Verification items for the finished model (mm, model axes). Coordinates: 2 decimals unless noted, no trailing zeros. Write each loop counter-clockwise with the first axis right and the second up, starting at its lowest first coordinate (ties: lowest second). Pieces come first, ordered by that corner, then holes. Notation, with made-up numbers: (2.5, 79.5) -> (60.5, 79.5) arc R28 cw to (60.5, 102.5) -> close; hole circle Ø6 at (-21.75, 78.5). An arc over 180 degrees is marked (long way). Answer in a Markdown table with one row per item.
```python
from build123d import *

# Parameters (mm, degrees)
SKETCH_W     = 42.3
SKETCH_H     = 42.3
SKETCH_R     = 11
PAD_DEPTH    = 2
CHAMFER_SIZE = 3.535534
SKETCH001_R  = 1.5
POCKET_DEPTH = 2.001


with BuildPart() as part:
    # Sketch → Pad (new body)
    with BuildSketch(Plane.XY):
        Rectangle(SKETCH_W, SKETCH_H)
        Circle(SKETCH_R, mode=Mode.SUBTRACT)
    extrude(amount=PAD_DEPTH)

    # Chamfer
    chamfer_edges = [part.edges().sort_by_distance(p)[0] for p in [
        (21.15, -21.15, 1),
        (21.15, 21.15, 1),
        (-21.15, -21.15, 1),
        (-21.15, 21.15, 1),
    ]]
    chamfer(chamfer_edges, length=CHAMFER_SIZE)

    # Sketch001 (on Face5 of Chamfer) → Pocket (cut, through all)
    with BuildSketch(Plane.XY.offset(2)):
        with Locations((15.5, 15.5)):
            Circle(SKETCH001_R)
        with Locations((-15.5, -15.5)):
            Circle(SKETCH001_R)
        with Locations((15.5, -15.5)):
            Circle(SKETCH001_R)
        with Locations((-15.5, 15.5)):
            Circle(SKETCH001_R)
    extrude(amount=-POCKET_DEPTH, mode=Mode.SUBTRACT)


solid = part.part
```
1. Sectioned sample at C-C, the plane z = 1.35. Record the cut outline in (x, y).
Findings below:
| item | result |
|---|---|
| outline | (-21.15, -17.61) -> (-17.61, -21.15) -> (17.61, -21.15) -> (21.15, -17.61) -> (21.15, 17.61) -> (17.61, 21.15) -> (-17.61, 21.15) -> (-21.15, 17.61) -> close; hole circle Ø3 at (-15.5, -15.5); hole circle Ø3 at (-15.5, 15.5); hole circle Ø22 at (0, 0); hole circle Ø3 at (15.5, -15.5); hole circle Ø3 at (15.5, 15.5) |
2. Release check for a two-part mould opening along X. For faces 1 (the face through (-10, -9, 0)), 2 (the face through (-2.38, -10.74, 0.99)), 3 (the face through (-19.357, -19.407, 0.986)) record: released by +X, released by -X, zero draft, split by the parting line, or undercut.
Findings below:
| item | result |
|---|---|
| face 1 | zero draft |
| face 2 | undercut |
| face 3 | released by -X |
3. Sectioned sample at B-B, the plane y = 0. Record the cut outline in (x, z).
Findings below:
| item | result |
|---|---|
| outline | (-21.15, 0) -> (-11, 0) -> (-11, 2) -> (-21.15, 2) -> close; (11, 0) -> (21.15, 0) -> (21.15, 2) -> (11, 2) -> close |
4. Material ranges on probe 1 along Y at (x, z) = (15.5, 1.6); probe 2 along X at (y, z) = (16, 1.05); probe 3 along Y at (x, z) = (0, 1.1), recorded low to high. Write a range as from..to.
Findings below:
| item | result |
|---|---|
| probe 1 | y = -21.15..-17, -14..14, 17..21.15 |
| probe 2 | x = -21.15..-16.91, -14.09..14.09, 16.91..21.15 |
| probe 3 | y = -21.15..-11, 11..21.15 |
5. Sectioned sample at A-A, the plane y = -15.5. Record the cut outline in (x, z), and give its area (3 significant figures).
Findings below:
| item | result |
|---|---|
| outline | (-21.15, 0) -> (-17, 0) -> (-17, 2) -> (-21.15, 2) -> close; (-14, 0) -> (14, 0) -> (14, 2) -> (-14, 2) -> close; (17, 0) -> (21.15, 0) -> (21.15, 2) -> (17, 2) -> close |
| area | 72.6 mm² |
6. Go/stop test with a flat-tipped pin: pin 1 (1.8 mm diameter, centred on x = -15.5, y = 15.5, fed in from -Z). Record where the tip stops, or that it passes through.
Findings below:
| item | result |
|---|---|
| pin 1 | passes through |
